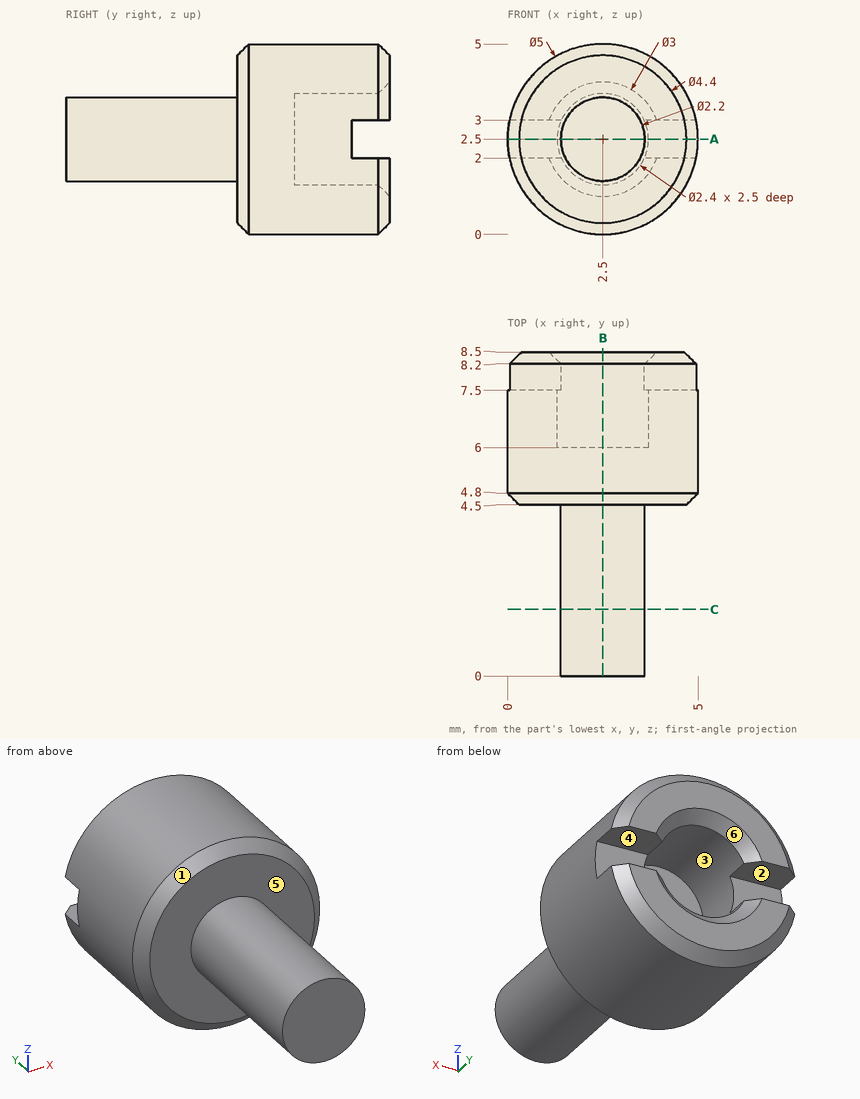
Job drawing, mm, ordinate dimensions from the low corner. One solid piece. A direction names the side the tool comes from. Coordinates: 2 decimals unless noted, no trailing zeros. Write each loop counter-clockwise with the first axis right and the second up, starting at its lowest first coordinate (ties: lowest second). Pieces come first, ordered by that corner, then holes.
Item 1: Mould opens along X. For the marked faces 1, 2 and 3 say: released by +X, released by -X, zero draft, split by the parting line, or undercut.
Item 2: Slice it at C-C (y = 1.75). Write the cut outline in (x, z).
Item 3: Probe line 1 (Z direction, x = 2.5, y = 7.05); line 2 (X direction, y = 3.5, z = 2.5). List the from-to ranges inside material, lowest first.
Item 4: Which spindle directions (+Z, -Z, +X, -X, +Y, -Y) get a long thin tool onto all of the face, cutting with end or side? Do the marked faces 4, 5 and 6. Say none if no direction does.
Item 5: Slice it at A-A (z = 2.5). Write the cut outline in (x, y), and give its area (3 significant figures).
Item 6: Pin check, flat tips, straight feed: pin 1 (1.2 mm diameter, centred on x = 3, z = 2.5, fed in from +Y); pin 2 (1.9 mm diameter, centred on x = 2.5, z = 2.5, fed in from -Y); pin 3 (0.5 mm diameter, centred on x = 0.5, y = 8, fed in from +Z); pin 4 (0.5 mm diameter, centred on x = 4, y = 8, fed in from +Z). Stop position of each tip, or through.
Item 7: Slice it at B-B (x = 2.5). Write the cut outline in (y, z).
Results found:
1. face 1: split by the parting line
1. face 2: zero draft
1. face 3: undercut
2. outline: circle Ø2.2 at (2.5, 2.5)
3. line 1: z = 0 to 1.3, 3.7 to 5
3. line 2: x = 1.4 to 3.6
4. face 4: +X, -X, +Y
4. face 5: -Y
4. face 6: +Y
5. outline: (0, 4.8) - (0.3, 4.5) - (1.4, 4.5) - (1.4, 0) - (3.6, 0) - (3.6, 4.5) - (4.7, 4.5) - (5, 4.8) - (5, 7.5) - (3.7, 7.5) - (3.7, 6) - (1.3, 6) - (1.3, 7.5) - (0, 7.5) - close
5. area: 21.2 mm2
6. pin 1: stops at y = 6
6. pin 2: stops at y = 0
6. pin 3: stops at z = 4.29
6. pin 4: stops at z = 4.67
7. outline: (0, 1.4) - (4.5, 1.4) - (4.5, 0.3) - (4.8, 0) - (8.2, 0) - (8.5, 0.3) - (8.5, 1) - (8.2, 1.3) - (6, 1.3) - (6, 3.7) - (8.2, 3.7) - (8.5, 4) - (8.5, 4.7) - (8.2, 5) - (4.8, 5) - (4.5, 4.7) - (4.5, 3.6) - (0, 3.6) - close
